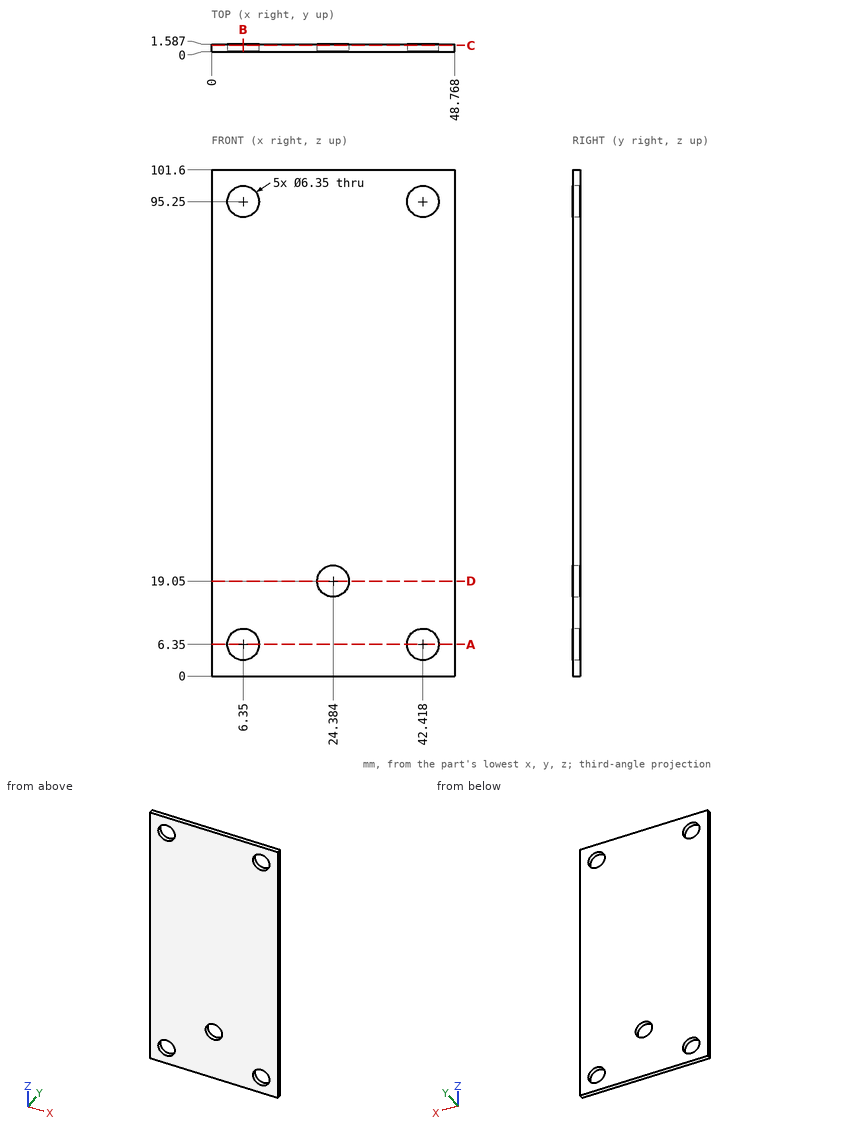
Drawing for the job (mm, zero at the part's lowest x, y, z). Round coordinates to 2 decimals unless told otherwise and drop trailing zeros. Loops run counter-clockwise (first coordinate to the right, second up) from the corner with the lowest first, then second, coordinate; pieces in that order, holes last. Notation, with made-up numbers: (16, 43) -> (62, 43) arc R24 ccw to (62, 61) -> close; hole circle Ø9 at (16, 40.5). An arc over 180 degrees is marked (long way). Answer in a Markdown table with one row per item.
Item 1: Saw through at A-A (z = 6.35). Write the cut outline in (x, y) (1 decimal).
Answers below:
| item | result |
|---|---|
| outline | (0, 0) -> (3.2, 0) -> (3.2, 1.6) -> (0, 1.6) -> close; (9.5, 0) -> (39.2, 0) -> (39.2, 1.6) -> (9.5, 1.6) -> close; (45.6, 0) -> (48.8, 0) -> (48.8, 1.6) -> (45.6, 1.6) -> close |
Item 2: Pin check, flat tip, straight feed: pin 1 (4 mm diameter, centred on x = 42.418, z = 95.25, fed in from +Y). Stop position of the tip, or through.
Answers below:
| item | result |
|---|---|
| pin 1 | passes through |
Item 3: Drill centre lines: L1, parallel to Z at x = 6.35, y = 0.5 (1 decimal); L2, parallel to X at y = 1.35, z = 95.25 (1 decimal); L3, parallel to X at y = 1.4, z = 97 (1 decimal). Where is each one in solid material? Low to high. Write a range as [from, to].
Answers below:
| item | result |
|---|---|
| L1 | z = [0, 3.2], [9.5, 92.1], [98.4, 101.6] |
| L2 | x = [0, 3.2], [9.5, 39.2], [45.6, 48.8] |
| L3 | x = [0, 3.7], [9, 39.8], [45.1, 48.8] |
Item 4: Saw through at D-D (z = 19.05). Write the cut outline in (x, y).
Answers below:
| item | result |
|---|---|
| outline | (0, 0) -> (21.21, 0) -> (21.21, 1.59) -> (0, 1.59) -> close; (27.56, 0) -> (48.77, 0) -> (48.77, 1.59) -> (27.56, 1.59) -> close |
Item 5: Saw through at C-C (y = 1.3). State how many separate pieces and enclosed holes the cut face has, and give its area (3 significant figures).
Answers below:
| item | result |
|---|---|
| separate pieces | 1 |
| enclosed holes | 5 |
| area | 4,800 mm² |
Item 6: Saw through at B-B (x = 6.35). Write the cut outline in (y, z) (1 decimal).
Answers below:
| item | result |
|---|---|
| outline | (0, 0) -> (1.6, 0) -> (1.6, 3.2) -> (0, 3.2) -> close; (0, 9.5) -> (1.6, 9.5) -> (1.6, 92.1) -> (0, 92.1) -> close; (0, 98.4) -> (1.6, 98.4) -> (1.6, 101.6) -> (0, 101.6) -> close |
